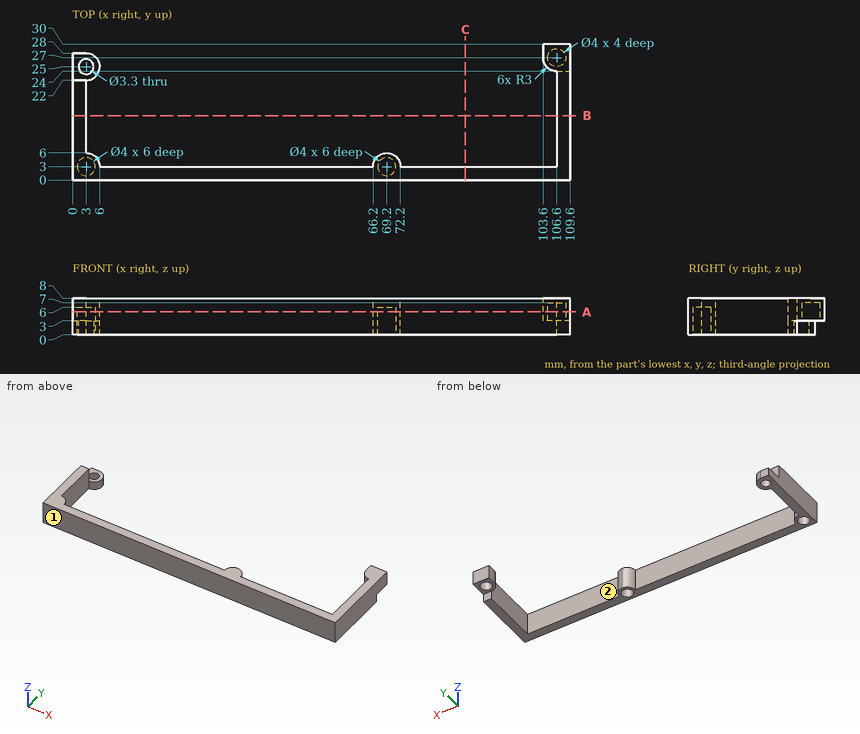
Input: dimensioned drawing with shaded views. Units: mm. Origin: part minimum x, y, z. Coordinates: 2 decimals unless noted, no trailing zeros. Order: outer loops, then holes, each group sorted by start corner. A loop starts at its lowest first (then second) coordinate and runs counter-clockwise, first axis right, second up. Notation, with made-up numbers: (60, 64.25) - (81, 64.25) arc R22 cw to (81, 88.25) - close; hole circle Ø9 at (2.5, 72.5). An arc over 180 degrees is marked (long way). One line per item, written item: value.
1) Cut plane A-A on z = 5. State how many separate pieces and enclosed holes the cut face has, plus the area to 3 significant figures.
Computed values:
separate pieces: 1
enclosed holes: 3
area: 466 mm^2
2) Ray query, line 1 (Y direction, x = 69.2, z = 2.4); line 2 (X direction, y = 6.25, z = 1); line 3 (X direction, y = 2.5, z = 5.5). Return the intervals inside material, ascending. Write a range as [from, to].
Computed values:
line 1: y = [0, 1], [5, 6]
line 2: x = [0, 3], [106.6, 109.6]
line 3: x = [0, 1.06], [4.94, 67.26], [71.14, 109.6]
3) Cut plane C-C on x = 86.5. Output: boundary loops of the cut face in (y, z).
Computed values:
outline: (0, 0) - (3, 0) - (3, 8) - (0, 8) - close
4) Cut plane B-B on y = 14.25. Output: boundary loops of the cut face in (x, z).
Computed values:
outline: (0, 0) - (3, 0) - (3, 8) - (0, 8) - close; (106.6, 0) - (109.6, 0) - (109.6, 8) - (106.6, 8) - close
5) Mould query, pull axis X, two halves, no side actions, for the marked faces 1 and 2. Classes: released by +X, released by -X, zero draft, split by the parting line, or undercut.
Computed values:
face 1: zero draft
face 2: undercut
6) Contact query for flat-ended pins moving along their axis: pin 1 (0.9 mm diameter, centred on x = 1.5, z = 6.5, fed in from +Y); pin 2 (5 mm diameter, centred on x = 107.5, y = 27, fed in from -Z); pin 3 (1.5 mm diameter, centred on x = 107.5, z = 1.5, fed in from +Y). Output: stop coordinate, or through.
Computed values:
pin 1: stops at y = 22
pin 2: stops at z = 3
pin 3: stops at y = 24
